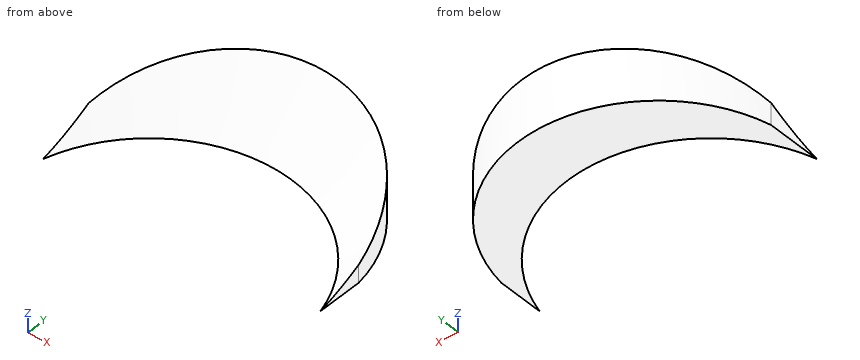
from build123d import *

# Parameters (mm, degrees)
F0_W        = 206.9673240185
F0_H        = 93.9061716199
F1_DEPTH    = 38.1
F3_DEPTH    = 38.1
F4_DEPTH    = 38.1
F5_T4_ANGLE = 333.9674626616
F6_W        = 206.9673240185
F6_H        = 38.1
F8_DEPTH    = 152.4


# Not quite as in the source:
# - a fillet or chamfer that OpenCascade refuses, or shapes differently, is made with other operations: its cross-section is extruded or revolved along the edge and cut away or added


with BuildPart() as f1:
    # F0 (on Top) → F1 (new body)
    with BuildSketch(Plane.XY):
        with Locations((-103.4836620092, 46.9530858099)):
            Rectangle(F0_W, F0_H)
    extrude(amount=F1_DEPTH)

    # F2 (on face) → F3 (join)
    with BuildSketch(Plane.XY.offset(38.1)):
        with BuildLine():
            Line((-38.5484881699, 19.2711967975), (-38.5484881699, 38.0954556167))
            ThreePointArc((-38.5484881699, 38.0954556167), (-95.9617823939, 88.596121937), (-155.8515280485, 41.0585366189))
            Line((-155.8515280485, 41.0585366189), (-155.8515280485, 19.9683923274))
            ThreePointArc((-155.8515280485, 19.9683923274), (-96.8534760925, 77.9237526804), (-38.5484881699, 19.2711967975))
        make_face()
    extrude(amount=F3_DEPTH)

    # F2 (on face) → F4 (join)
    with BuildSketch(Plane.XY.offset(38.1)):
        with BuildLine():
            ThreePointArc((-155.8515280485, 18.5740012676), (-97.4655811383, 63.6052200178), (-38.5484881699, 19.2711967975))
            ThreePointArc((-38.5484881699, 19.2711967975), (-96.8534760925, 77.9237526804), (-155.8515280485, 19.9683923274))
            Line((-155.8515280485, 19.9683923274), (-155.8515280485, 18.5740012676))
        make_face()
    extrude(amount=F4_DEPTH)

    # F5: chamfer of 38.1 on 1 edges, made by hand


with BuildPart() as f5_tool2:
    # F5_s3 → F5_t4 (revolve)
    with BuildSketch(Plane(origin=(-93.0214210663, 20.9218871248, 0), x_dir=(0, 0, 1), z_dir=(0.9756275706, -0.2194330045, 0))):
        Polygon((38.1, 79.4412595984), (76.2, 117.5412595984), (76.2, 79.4412595984), align=None)
    revolve(axis=Axis((-97.1040055743, 2.7701874098, 76.2), (0, 0, -1)), revolution_arc=F5_T4_ANGLE)

    split(bisect_by=Plane.XY.offset(38.1), keep=Keep.TOP)


with BuildPart() as f1_1:
    add(f1.part)

    # F5_t1: cut F5_tool2
    add(f5_tool2.part, mode=Mode.SUBTRACT)

    # F6 (on face) → F8 (cut)
    with BuildSketch(Plane.XZ):
        with Locations((-103.4836620092, 19.05)):
            Rectangle(F6_W, F6_H)
    extrude(amount=-F8_DEPTH, mode=Mode.SUBTRACT)


solid = f1_1.part
Verification items for the finished model (mm, model axes). Coordinates: 2 decimals unless noted, no trailing zeros. Order: outer loops, then holes, each group sorted by start corner. A loop starts at its lowest first (then second) coordinate and runs counter-clockwise, first axis right, second up.
1. Sectioned sample at A-A, the plane z = 42.5. Record the cut outline in (x, y), and give its area (3 significant figures).
Results found:
outline: (-155.85, 31.13) arc R65.24 cw to (-38.55, 31.53) - (-38.55, 38.1) arc R59.62 ccw to (-155.85, 41.06) - close
area: 2,210 mm2
2. Scan lines: line 1 (X direction, y = 51, z = 49); line 2 (X direction, y = 37, z = 42.75); line 3 (Y direction, x = -131, z = 48.5). Record each from-to range of solid material in increasing order.
Results found:
line 1: x = -152.88 to -150.21, -44 to -42.06
line 2: x = -155.85 to -152.93, -41.28 to -38.55
line 3: y = 65.43 to 78.29
3. Go/stop test with flat-tipped pins: pin 1 Ø8 at (y, z) = (72, 45.5) entering from +X; pin 2 Ø4 at (x, z) = (-136, 41.5) entering from -Y; pin 3 Ø6 at (x, z) = (-69, 59.5) entering from +Y. Record where each tip stops, or that it passes through.
Results found:
pin 1: stops at x = -52.38
pin 2: stops at y = 50.88
pin 3: stops at y = 82.9
4. Sectioned sample at B-B, the plane z = 56.5. Record the cut outline in (x, y).
Results found:
outline: (-143.25, 67.18) arc R79.24 cw to (-52.76, 68.43) arc R59.62 ccw to start
